from build123d import *

# Parameters (mm, degrees)
ENL_V_MAT_EXTRU_1_DEPTH = 1
CHANFREIN1_SIZE         = 0.2
CONG_1_R                = 0.2
CONG_2_R                = 0.2


# Read off the part's stored shape, not the designer's step: M2.5 Filetages mécaniques Borne3
with BuildPart() as part:
    # Esquisse1 → Révolution1 (revolve)
    with BuildSketch(Plane.XY):
        with BuildLine():
            Line((0, 0), (-9, 0))
            ThreePointArc((-9, 0), (-8.873105626, 1.030776406), (-8.5, 2))
            Line((-8.5, 2), (-8, 2))
            Line((-8, 2), (-8, 1.5))
            Line((-8, 1.5), (0, 1.5))
            Line((0, 1.5), (0, 0))
        make_face()
    revolve(axis=Axis((0, 0, 0), (-1, 0, 0)))

    # Esquisse2 → Enlèv. mat.-Extru.1 (cut)
    with BuildSketch(Plane.ZY.offset(9)):
        Polygon((-0.25, 1.25), (0.25, 1.25), (0.25, 0.25), (1.25, 0.25), (1.25, -0.25), (0.25, -0.25), (0.25, -1.25), (-0.25, -1.25), (-0.25, -0.25), (-1.25, -0.25), (-1.25, 0.25), (-0.25, 0.25), align=None)
    extrude(amount=-ENL_V_MAT_EXTRU_1_DEPTH, mode=Mode.SUBTRACT)

    # Chanfrein1
    chanfrein1_edges = [part.edges().sort_by_distance(p)[0] for p in [
        (-8.492634293, 0.25, 0.25),
        (-8.492634293, -0.25, 0.25),
        (-8.492634293, -0.25, -0.25),
        (-8.492634293, 0.25, -0.25),
    ]]
    chamfer(chanfrein1_edges, length=CHANFREIN1_SIZE)

    # Enlèv. mat.-Extru.3 cone 1 section (through the dimple's axis) → Enlèv. mat.-Extru.3 (revolve, cut)
    with BuildSketch(Plane(origin=(-8, 0, 0), x_dir=(0, 0, 1), z_dir=(0, 1, 0))):
        Polygon((0, 0), (0.494974747, 0), (0, 0.043304679), align=None)
    revolve(axis=Axis((-8, 0, 0), (1, 0, 0)), mode=Mode.SUBTRACT)

    # Congé1
    cong_1_edges = [part.edges().sort_by_distance(p)[0] for p in [
        (-8, -1.5, 0),
    ]]
    fillet(cong_1_edges, radius=CONG_1_R)

    # Congé2
    cong_2_edges = [part.edges().sort_by_distance(p)[0] for p in [
        (-8.5, -2, 0),
    ]]
    fillet(cong_2_edges, radius=CONG_2_R)

    # M2.5 Filetages mécaniques Borne3 outline → M2.5 Filetages mécaniques Borne3 (revolve, cut)
    with BuildSketch(Plane.YX):
        Polygon((1.5, 0), (0.9965, 0), (1.25, -0.2535), (1.25, -7.8), (1.5, -7.8), align=None)
    revolve(axis=Axis((0, 0, 0), (1, 0, 0)), mode=Mode.SUBTRACT)


solid = part.part
The listing builds one solid part. Answer for the finished solid, in the listing's coordinates (mm). A direction names the side the tool comes from. Coordinates: 2 decimals unless noted, no trailing zeros. Order: outer loops, then holes, each group sorted by start corner. A loop starts at its lowest first (then second) coordinate and runs counter-clockwise, first axis right, second up. Notation, with made-up numbers: M 85,59.5 L 133,59.5 A22 cw 133,85.5 Z; hole C 65.25,47.5 d1. An arc over 180 degrees is marked long. Use CSV: the item, a comma, the result in double quotes.
Q1. Straight lines are drawn through the part: L1, parallel to X at y = -0.05, z = 0.5; L2, parallel to Z at x = -1.5, y = 0.05; L3, parallel to X at y = 1.1, z = 0.3. For each, find the intervals that lie inside material, in ascending order.
Here are the results:
L1,"-8 to 0"
L2,"-1.25 to 1.25"
L3,"-8.84 to -0.14"
Q2. A tool of negligible diameter and unlimited length cuts with its end or side. For faces 4 (the cylindrical face through (-8.186, 1.908, -0.601)), 5 (the flat face through (-8.5, -0.8, 0.25)), from which of +Z, -Z, +X, -X, +Y, -Y can it reach the whole face along a straight path? Write none if from no direction.
Here are the results:
face 4,"+X, -X"
face 5,"-X"
Q3. Given pin 1 Ø1 at (x, z) = (-1.5, 1) entering from -Y; pin 2 Ø0.6 at (x, y) = (-8.5, -1) entering from +Z; pin 3 Ø0.6 at (x, z) = (-8.5, 1) entering from -Y, each flat-ended and moving along its own axis, determine where each tip first touches the part or whether it passes through.
Here are the results:
pin 1,"y = -1.15"
pin 2,"z = 1.87"
pin 3,"y = -1.87"
Q4. Determine the mould class of faces 1 (the cylindrical face through (-4.08, -0.27, -1.22)), 2 (the flat face through (0, 0, 0)), 3 (the flat face through (-8.5, 0.25, 0.8)) for opening direction Z: pulls with the +Z half, pulls with the -Z half, needs draft (parallel to the pull), parting line crosses it, or undercut.
Here are the results:
face 1,"parting line crosses it"
face 2,"needs draft"
face 3,"undercut"
Q5. Section A-A (x = -2.75) is taken. Determine the outline of the cut face in (y, z).
Here are the results:
outline,"C 0,0 d2.5"
